Geometry: see drawing. Coordinates: mm, zero at the bounding-box minimum. Give positions to 0.01 mm unless a question says otherwise; leave off trailing zeros. Write each loop counter-clockwise with the first axis right and the second up, starting at its lowest first coordinate (ties: lowest second). Pieces come first, ordered by that corner, then holes. Notation, with made-up numbers: M -22.75,25.5 L 4.25,25.5 A21 ccw 4.25,55.5 Z; hole C -28,70 d9. An arc over 180 degrees is marked long. Use a Markdown table: item, result. Add a question column.
1) Section A-A on x = 25. Return the cut outline in (y, z), then the cut area to 3 significant figures.
2) Pin query (flat end, axial travel): pin 1 (1.2 mm diameter, centred on x = 25, z = 12.5, fed in from +Y); pin 2 (0.9 mm diameter, centred on x = 28, y = 3, fed in from +Z). Return the tip coordinate at first contact, or that it passes through.
3) Line query: line 1 (X direction, y = 0.5, z = 12.5); line 2 (X direction, y = 4.9, z = 12.5); line 3 (X direction, y = 4.7, z = 11.75). Output: solid intervals per line, ascending.
4) Section C-C on x = 47. Return the cut outline in (y, z).
5) Draft query along Z for the marked faces 1 and 2. Return one class per face: +Z half, -Z half, draft (parallel to the pull), parting line (faces both ways), or undercut.
6) Section B-B on z = 12.5. State how many separate pieces and enclosed holes the cut face has, then the cut area to 3 significant figures.
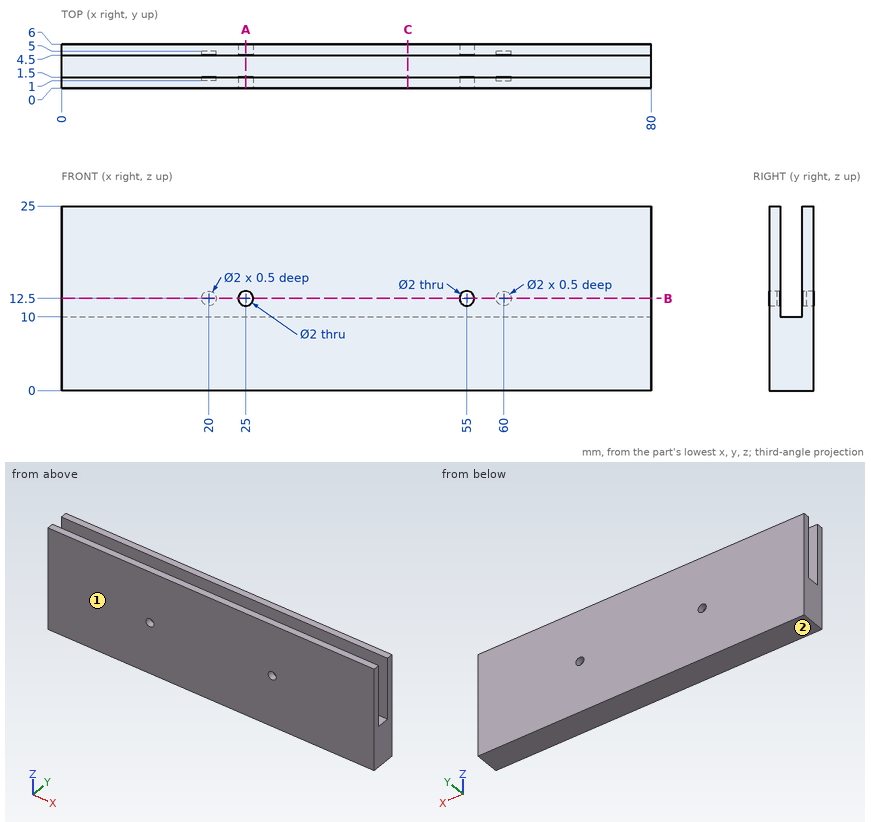
Found:
| question | item | result |
|---|---|---|
| 1 | outline | M 0,0 L 6,0 L 6,11.5 L 4.5,11.5 L 4.5,10 L 1.5,10 L 1.5,11.5 L 0,11.5 Z; M 0,13.5 L 1.5,13.5 L 1.5,25 L 0,25 Z; M 4.5,13.5 L 6,13.5 L 6,25 L 4.5,25 Z |
| 1 | area | 99.0 mm² |
| 2 | pin 1 | through |
| 2 | pin 2 | z = 10 |
| 3 | line 1 | 0 to 24, 26 to 54, 56 to 80 |
| 3 | line 2 | 0 to 19, 21 to 24, 26 to 54, 56 to 59, 61 to 80 |
| 3 | line 3 | 0 to 19.34, 20.66 to 24.34, 25.66 to 54.34, 55.66 to 59.34, 60.66 to 80 |
| 4 | outline | M 0,0 L 6,0 L 6,25 L 4.5,25 L 4.5,10 L 1.5,10 L 1.5,25 L 0,25 Z |
| 5 | face 1 | draft |
| 5 | face 2 | -Z half |
| 6 | separate pieces | 6 |
| 6 | enclosed holes | 0 |
| 6 | area | 224 mm² |
